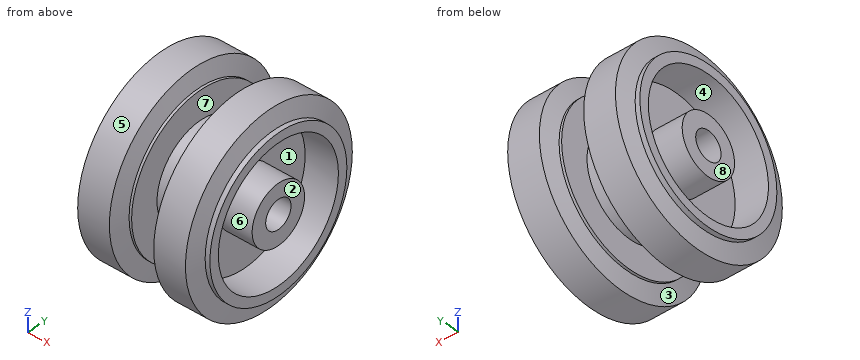
```python
from build123d import *

# Parameters (mm, degrees)
SKETCH2_W   = 10.5
SKETCH2_H   = 12
SKETCH2_W_2 = 15
SKETCH2_H_2 = 4.5


with BuildPart() as part:
    # Sketch1 → Revolve1 (revolve)
    with BuildSketch(Plane.XY):
        Polygon((0, 0), (0, 15.3), (-4.7, 15.3), (-4.7, 24.3), (-5.5, 24.3), (-7, 29.6), (-17, 29.6), (-18.5, 24.3), (-20, 24.3), (-20, 0), align=None)
    revolve1 = revolve(axis=Axis((-20, 0, 0), (1, 0, 0)))

    # Sketch2 → Cut-Revolve1 (revolve, cut)
    with BuildSketch(Plane.XY):
        with Locations((-14.75, 15.3)):
            Rectangle(SKETCH2_W, SKETCH2_H)
        with Locations((-12.5, 2.25)):
            Rectangle(SKETCH2_W_2, SKETCH2_H_2)
    cut_revolve1 = revolve(axis=Axis((0, 0, 0), (-1, 0, 0)), mode=Mode.SUBTRACT)

    # Mirror1: Revolve1, Cut-Revolve1 across plane
    add(revolve1.mirror(Plane.ZY))
    add(cut_revolve1.mirror(Plane.ZY), mode=Mode.SUBTRACT)


solid = part.part
```
Check sheet for the modelled part. Datum: model origin and axes. Units: mm. Face numbers are marked on the shaded views. A direction names the side the tool comes from. Give positions to 0.01 mm unless a question says otherwise; leave off trailing zeros. Write each loop counter-clockwise with the first axis right and the second up, starting at its lowest first coordinate (ties: lowest second). Pieces come first, ordered by that corner, then holes. Notation, with made-up numbers: (61.25, -23.75) -> (120.25, -23.75) arc R28 ccw to (120.25, 5.25) -> close; hole circle Ø8 at (-38, 48.25). An arc over 180 degrees is marked (long way). Use CSV: the item, a comma, the result in double quotes. Start each with the question number.
Q1. Cross-section at A-A on x = 14.5. Enter the section's corners in (y, z).
Q2. Tool access check on the marked faces 1, 2, 3, 4 and 5. Record the directions out of +Z, -Z, +X, -X, +Y, -Y that give a thin tool (end or side, any length) a straight path to the whole face; none if there is none.
Q3. Depth check by flat-ended pin: P1, Ø8, axis at y = 0, z = 0, coming from the +X side; P2, Ø8, axis at x = 5.5, y = 6.5, coming from the -Z side; P3, Ø4, axis at x = -15, y = -10, coming from the +Z side. Enter the tip coordinate at first touch or a pass-through.
Q4. Scan lines: line 1 along Z through (x, y) = (-16.25, 0); line 2 along X through (y, z) = (12, -27); line 3 along X through (y, z) = (-19, 1.5). Record each from-to range of solid material in increasing order.
Q5. Release check for a two-part mould opening along X. For the marked faces 6, 7 and 8 record: +X half, -X half, draft (parallel to the pull), parting line (faces both ways), or undercut.
Working result:
1,outline,"circle Ø59.2 at (0, 0); circle Ø18.6 at (0, 0); hole circle Ø42.6 at (0, 0); hole circle Ø9 at (0, 0)"
2,face 1,"+X"
2,face 2,"+Z, -Z, +X, +Y, -Y"
2,face 3,"none"
2,face 4,"-X"
2,face 5,"+X, -X"
3,P1,"stops at x = 5"
3,P2,"stops at z = -29.47"
3,P3,"stops at z = 28.5"
4,line 1,"z = -29.6 to -21.3, -9.3 to -4.5, 4.5 to 9.3, 21.3 to 29.6"
4,line 2,"x = -17.02 to -6.98, 6.98 to 17.02"
4,line 3,"x = -9.5 to -4.7, 4.7 to 9.5"
5,face 6,"draft"
5,face 7,"undercut"
5,face 8,"-X half"
